```python
from build123d import *

# Parameters (mm, degrees)
SKETCH1_R           = 11.938
SKETCH1_R_2         = 8.763
BOSS_EXTRUDE1_DEPTH = 5.08
SKETCH2_R           = 11.938
BOSS_EXTRUDE2_DEPTH = 2.54
BOSS_EXTRUDE5_DEPTH = 2.54


with BuildPart() as part:
    # Sketch1 → Boss-Extrude1 (new body)
    with BuildSketch(Plane.XY):
        Circle(SKETCH1_R)
        Circle(SKETCH1_R_2, mode=Mode.SUBTRACT)
    extrude(amount=BOSS_EXTRUDE1_DEPTH)

    # Sketch2 → Boss-Extrude2 (add)
    with BuildSketch(Plane.XY.offset(5.08)):
        Circle(SKETCH2_R)
    extrude(amount=BOSS_EXTRUDE2_DEPTH)

    # Sketch3 → Boss-Extrude5 (add)
    with BuildSketch(Plane.XY.offset(7.62)):
        with BuildLine():
            Line((-3.749775554, -5.025912703), (-3.749775554, -4.357730643))
            ThreePointArc((-3.749775554, -4.357730643), (-1.563899962, -2.052721882), (-1.176728716, 1.100247499))
            Line((-1.176728716, 1.100247499), (-3.294944042, -1.771688619))
            Line((-3.294944042, -1.771688619), (-5.621082346, -0.55014113))
            Line((-5.621082346, -0.55014113), (-5.062289346, 5.462731457))
            Line((-5.062289346, 5.462731457), (-5.621082346, 6.523138639))
            Line((-5.621082346, 6.523138639), (-0.422811908, 6.523138639))
            ThreePointArc((-0.422811908, 6.523138639), (2.824920532, 4.69173738), (3.826417915, 1.100247499))
            ThreePointArc((3.826417915, 1.100247499), (3.353249923, -1.024672289), (3.304473127, -3.20108973))
            ThreePointArc((3.304473127, -3.20108973), (3.557112423, -3.847120346), (3.826417915, -4.486382985))
            Line((3.826417915, -4.486382985), (3.826417915, -5.025912703))
            Line((3.826417915, -5.025912703), (4.519556937, -5.025912703))
            Line((4.519556937, -5.025912703), (4.519556937, -7.490281135))
            Line((4.519556937, -7.490281135), (-4.344219843, -7.490281135))
            Line((-4.344219843, -7.490281135), (-4.344219843, -5.025912703))
            Line((-4.344219843, -5.025912703), (-3.749775554, -5.025912703))
        make_face()
    extrude(amount=BOSS_EXTRUDE5_DEPTH)


solid = part.part
```
Part model, mm, in its own coordinate system. A direction names the side the tool comes from. Round coordinates to 2 decimals unless told otherwise and drop trailing zeros. Write each loop counter-clockwise with the first axis right and the second up, starting at its lowest first coordinate (ties: lowest second). Pieces come first, ordered by that corner, then holes.
Item 1: Probe L1, parallel to X at y = 0.25, z = 3.5; L2, parallel to Z at x = 2.5, y = -1. List the from-to ranges inside material, lowest first.
Results:
L1: x = -11.94 to -8.76, 8.76 to 11.94
L2: z = 5.08 to 10.16
Item 2: Cut at A-A, the plane z = 9. Give the cut face in (x, y), plus the area to 3 significant figures.
Results:
outline: (-5.62, -0.55) - (-3.29, -1.77) - (-1.18, 1.1) arc R5.07 cw to (-3.75, -4.36) - (-3.75, -5.03) - (-4.34, -5.03) - (-4.34, -7.49) - (4.52, -7.49) - (4.52, -5.03) - (3.83, -5.03) - (3.83, -4.49) arc R26.75 cw to (3.3, -3.2) arc R11.09 cw to (3.83, 1.1) arc R4.87 ccw to (-0.42, 6.52) - (-5.62, 6.52) - (-5.06, 5.46) - close
area: 108 mm2
Item 3: Cut at B-B, the plane x = -2.75. Give the cut face in (y, z), plus the area to 3 significant figures.
Results:
outline: (-11.62, 0) - (-8.32, 0) - (-8.32, 5.08) - (8.32, 5.08) - (8.32, 0) - (11.62, 0) - (11.62, 7.62) - (6.52, 7.62) - (6.52, 10.16) - (-1.03, 10.16) - (-1.03, 7.62) - (-3.65, 7.62) - (-3.65, 10.16) - (-7.49, 10.16) - (-7.49, 7.62) - (-11.62, 7.62) - close
area: 121 mm2
Item 4: Cut at C-C, the plane z = 4.25. Give the cut face in (x, y), plus the area to 3 significant figures.
Results:
outline: circle Ø23.88 at (0, 0); hole circle Ø17.53 at (0, 0)
area: 206 mm2
Item 5: Cut at D-D, the plane y = -7. Give the cut face in (x, z).
Results:
outline: (-9.67, 0) - (-5.27, 0) - (-5.27, 5.08) - (5.27, 5.08) - (5.27, 0) - (9.67, 0) - (9.67, 7.62) - (4.52, 7.62) - (4.52, 10.16) - (-4.34, 10.16) - (-4.34, 7.62) - (-9.67, 7.62) - close
Item 6: Drop flat-ended pins along their axis: pin 1 Ø2 at (x, z) = (5, 4.5) entering from -Y; pin 2 Ø0.7 at (y, z) = (-5, 9) entering from -X; pin 3 Ø0.8 at (x, z) = (-1, 8.5) entering from -Y; pin 4 Ø10 at (x, y) = (-5, -1.5) entering from -Z. Give the stop position or say it passes through.
Results:
pin 1: stops at y = -11.25
pin 2: stops at x = -4.34
pin 3: stops at y = -7.49
pin 4: stops at z = 0
Item 7: Which spindle directions (+Z, -Z, +X, -X, +Y, -Y) get a long thin tool onto all of the face, cutting with end or side? Do faces 4 (the flat face through (-4.44, -1.17, 8.87)), 5 (the cylindrical face through (8.36, 2.63, 2.5)), 6 (the cylindrical face through (3.553, -3.838, 8.872)), 7 (the flat face through (-4.344, -6, 9)). Say none if no direction does.
Results:
face 4: +Z, -X
face 5: -Z
face 6: +Z, +X
face 7: +Z, -X, -Y
Item 8: Two-plate mould, pull along Y, no slides. Class faces 1 (the flat face through (-3, 6.523, 9)), 2 (the flat face through (4.52, -6, 9)), 3 (the flat face through (-5.346, 2.414, 8.872)): +Y half, -Y half, draft (parallel to the pull), parting line (faces both ways), or undercut.
Results:
face 1: +Y half
face 2: draft
face 3: undercut
